Read the model definition and answer for the solid it produces. Units are mm, in the model's axes. A direction names the side the tool comes from. Coordinates: 2 decimals unless noted, no trailing zeros. Write each loop counter-clockwise with the first axis right and the second up, starting at its lowest first coordinate (ties: lowest second). Pieces come first, ordered by that corner, then holes. Notation, with made-up numbers: (59.5, 23) -> (105.5, 23) arc R26 ccw to (105.5, 39) -> close; hole circle Ø4 at (11.25, -20.75). An arc over 180 degrees is marked (long way). Answer in a Markdown table with one row per item. Add a question column.
Item 1: Section D-D on z = 0.8 is taken. Count the separate pieces of the cut face and the enclosed holes in it, then the cut area to 3 significant figures.
Item 2: Section B-B on x = -5 is taken. Write down the section's boundary in (y, z).
Item 3: Section A-A on y = -24.5 is taken. Write down the section's boundary in (x, z).
Item 4: Which of the six approach directions +Z, -Z, +X, -X, +Y, -Y give full straight-line access (tool end or side, diameter ignored) to faces 1 (the face through (32, -30.75, 1)), 2 (the face through (29, 19.75, 1)), 3 (the face through (0, 13.5, 1)), 4 (the face through (27.25, -26, 1))?
Item 5: Section C-C on y = 15.5 is taken. Write down the section's boundary in (x, z).
Item 6: Given pin 1 Ø3 at (x, y) = (-16, 7.5) entering from -Z; pin 2 Ø0.9 at (x, z) = (29.5, 1) entering from -Y; pin 3 Ø1.5 at (x, z) = (29, 1) entering from +Y, each flat-ended and moving along its own axis, determine where each tip first touches the part or whether it passes through.
Item 7: Straight lines are drawn through the part: line 1 (Y direction, x = 29, z = 1.9); line 2 (X direction, y = 15.5, z = 0.5); line 3 (Y direction, x = -28.5, z = 0.3). For each, find the intervals that lie inside material, in ascending order. Write a range as from..to.
Item 8: For a pull along Y with two mould halves and no side action, classify faces 5 (the face through (29, 4, 1)), 6 (the face through (0, 0, 3)), 7 (the face through (30.75, -9, 1)), 8 (the face through (-3, -30.75, 1)) as +Y half, -Y half, draft (parallel to the pull), parting line (faces both ways), or undercut.
```python
from build123d import *

# Parameters (mm, degrees)
SKETCH_1_W      = 15.5
SKETCH_1_H      = 3.5
SKETCH_1_W_2    = 10.5
SKETCH_1_W_3    = 3.5
SKETCH_1_H_2    = 5.5
SKETCH_1_H_3    = 10.5
EXTRUDE_1_DEPTH = 3


with BuildPart() as part:
    # Эскиз1 → Бобышка-Вытянуть1 (new body)
    with BuildSketch(Plane.XY):
        Polygon((30.75, -30.75), (33, -30.75), (33, 30.25), (30.75, 30.25), (30.75, 19.75), (27.25, 19.75), (27.25, 30.25), (-33, 30.25), (-33, -30.75), (27.25, -30.75), (27.25, -21.25), (30.75, -21.25), align=None)
        Polygon((-27.25, 13.25), (-27.25, 9.25), (-30.75, 9.25), (-30.75, 19.75), (-27.25, 19.75), (-27.25, 16.75), (-17, 16.75), (-17, 13.25), align=None, mode=Mode.SUBTRACT)
        with Locations((-0.25, 15.25)):
            Rectangle(SKETCH_1_W, SKETCH_1_H, mode=Mode.SUBTRACT)
        with Locations((21.75, 15.25)):
            Rectangle(SKETCH_1_W_2, SKETCH_1_H, mode=Mode.SUBTRACT)
        with Locations((29, 6.75)):
            Rectangle(SKETCH_1_W_3, SKETCH_1_H_2, mode=Mode.SUBTRACT)
        with Locations((29, -9)):
            Rectangle(SKETCH_1_W_3, SKETCH_1_H_2, mode=Mode.SUBTRACT)
        with Locations((-29, -0.5)):
            Rectangle(SKETCH_1_W_3, SKETCH_1_H_3, mode=Mode.SUBTRACT)
        with Locations((-29, -15.25)):
            Rectangle(SKETCH_1_W_3, SKETCH_1_H_3, mode=Mode.SUBTRACT)
    extrude(amount=EXTRUDE_1_DEPTH)


solid = part.part
```
Results below:
| question | item | result |
|---|---|---|
| 1 | separate pieces | 1 |
| 1 | enclosed holes | 7 |
| 1 | area | 3,680 mm2 |
| 2 | outline | (-30.75, 0) -> (13.5, 0) -> (13.5, 3) -> (-30.75, 3) -> close; (17, 0) -> (30.25, 0) -> (30.25, 3) -> (17, 3) -> close |
| 3 | outline | (-33, 0) -> (27.25, 0) -> (27.25, 3) -> (-33, 3) -> close; (30.75, 0) -> (33, 0) -> (33, 3) -> (30.75, 3) -> close |
| 4 | face 1 | +Z, -Z, +X, -X, -Y |
| 4 | face 2 | +Z, -Z, +Y |
| 4 | face 3 | +Z, -Z |
| 4 | face 4 | +Z, -Z, -Y |
| 5 | outline | (-33, 0) -> (-30.75, 0) -> (-30.75, 3) -> (-33, 3) -> close; (-17, 0) -> (-8, 0) -> (-8, 3) -> (-17, 3) -> close; (7.5, 0) -> (16.5, 0) -> (16.5, 3) -> (7.5, 3) -> close; (27, 0) -> (33, 0) -> (33, 3) -> (27, 3) -> close |
| 6 | pin 1 | stops at z = 0 |
| 6 | pin 2 | stops at y = -21.25 |
| 6 | pin 3 | stops at y = 19.75 |
| 7 | line 1 | y = -21.25..-11.75, -6.25..4, 9.5..19.75 |
| 7 | line 2 | x = -33..-30.75, -17..-8, 7.5..16.5, 27..33 |
| 7 | line 3 | y = -30.75..-20.5, -10..-5.75, 4.75..9.25, 19.75..30.25 |
| 8 | face 5 | undercut |
| 8 | face 6 | draft |
| 8 | face 7 | undercut |
| 8 | face 8 | -Y half |
